Geometry: final body of the model. Coordinates: model frame, mm. A direction names the side the tool comes from. Give positions to 0.01 mm unless a question says otherwise; leave off trailing zeros. Write each loop counter-clockwise with the first axis right and the second up, starting at its lowest first coordinate (ties: lowest second). Pieces come first, ordered by that corner, then holes. Notation, with made-up numbers: M 37,51.5 L 90,51.5 A22 ccw 90,71.5 Z; hole C 74,77 d9. An arc over 180 degrees is marked long. Use a Markdown table: item, result. Add a question column.
(1) Draft query along X for faces 1 (the flat face through (0, 1, -23)), 2 (the flat face through (42, 0, -28)), 3 (the flat face through (72.4, 1, -42)). Return one class per face: released by +X, released by -X, zero draft, split by the parting line, or undercut.
(2) Pin query (flat end, axial travel): pin 1 Ø0.6 at (x, y) = (11.5, 1) entering from +Z; pin 2 Ø1.8 at (x, z) = (77.4, -42.5) entering from +Y (1 decimal). Return the tip coordinate at first contact, or that it passes through.
(3) Cut plane D-D (y = 1.35). State how many separate pieces and enclosed holes the cut face has, plus the area to 3 significant figures.
(4) Reachability of faces 4 (the flat face through (82.4, 1, -3)), 5 (the flat face through (4, 1, -43)), 6 (the flat face through (83, 1, -45)) from +Z, -Z, +X, -X, +Y, -Y: full face, straight path, thin tool, end or side. Return the list, or none.
(5) Cut plane C-C (x = 44). Output: boundary loops of the cut face in (y, z).
(6) Cut plane A-A (x = 77.4). Output: boundary loops of the cut face in (y, z), plus the area to 3 significant figures.
(7) Cut plane B-B (z = -42.5). Output: boundary loops of the cut face in (x, y), plus the area to 3 significant figures.
(8) Material intervals for L1, parallel to Z at x = 77.4, y = 1.05; L2, parallel to X at y = 1.1, z = -23; L3, parallel to X at y = 0.1, z = -24, sorted ascending.
```python
from build123d import *

# Parameters (mm, degrees)
SKETCH1_R           = 1.5
BOSS_EXTRUDE1_DEPTH = 2
SKETCH2_W           = 8.75
SKETCH2_H           = 3.4
CUT_EXTRUDE1_DEPTH  = 10
FILLET1_R           = 1.3


with BuildPart() as part:
    # Sketch1 → Boss-Extrude1 (new body)
    with BuildSketch(Plane(origin=(0, 0, 0), x_dir=(1, 0, 0), z_dir=(0, 1, 0))):
        Polygon((0, 0), (2, 0), (2, 5), (4, 5), (4, 0), (10, 0), (10, 5), (12, 5), (12, 0), (72.4, 0), (72.4, 5), (74.4, 5), (74.4, 0), (80.4, 0), (80.4, 5), (82.4, 5), (82.4, 0), (84.4, 0), (84.4, 45), (82.4, 45), (82.4, 40), (80.4, 40), (80.4, 45), (74.4, 45), (74.4, 40), (72.4, 40), (72.4, 45), (12, 45), (12, 40), (10, 40), (10, 45), (4, 45), (4, 40), (2, 40), (2, 45), (0, 45), align=None)
        with Locations(Location((7, 42.5, 0), (0, 0, 270))):
            Circle(SKETCH1_R, mode=Mode.SUBTRACT)
        with Locations(Location((77.4, 42.5, 0), (0, 0, 90))):
            Circle(SKETCH1_R, mode=Mode.SUBTRACT)
        with Locations(Location((7, 2.5, 0), (0, 0, 90))):
            Circle(SKETCH1_R, mode=Mode.SUBTRACT)
        with Locations(Location((77.4, 2.5, 0), (0, 0, 270))):
            Circle(SKETCH1_R, mode=Mode.SUBTRACT)
    extrude(amount=BOSS_EXTRUDE1_DEPTH)

    # Sketch2 → Cut-Extrude1 (cut)
    with BuildSketch(Plane(origin=(0, 2, 0), x_dir=(1, 0, 0), z_dir=(0, 1, 0))):
        with Locations((42.2, 22.5)):
            Rectangle(SKETCH2_W, SKETCH2_H)
    extrude(amount=-CUT_EXTRUDE1_DEPTH, mode=Mode.SUBTRACT)

    # Fillet1
    fillet1_edges = [part.edges().sort_by_distance(p)[0] for p in [
        (46.575, 1, -24.2),
        (46.575, 1, -20.8),
        (37.825, 1, -20.8),
        (37.825, 1, -24.2),
    ]]
    fillet(fillet1_edges, radius=FILLET1_R)


solid = part.part
```
Answer list:
| question | item | result |
|---|---|---|
| 1 | face 1 | released by -X |
| 1 | face 2 | zero draft |
| 1 | face 3 | undercut |
| 2 | pin 1 | z = -5 |
| 2 | pin 2 | through |
| 3 | separate pieces | 1 |
| 3 | enclosed holes | 5 |
| 3 | area | 3,660 mm² |
| 4 | face 4 | +Z, +Y, -Y |
| 4 | face 5 | -Z, +Y, -Y |
| 4 | face 6 | -Z, +X, -X, +Y, -Y |
| 5 | outline | M 0,-45 L 2,-45 L 2,-24.2 L 0,-24.2 Z; M 0,-20.8 L 2,-20.8 L 2,0 L 0,0 Z |
| 6 | outline | M 0,-45 L 2,-45 L 2,-44 L 0,-44 Z; M 0,-41 L 2,-41 L 2,-4 L 0,-4 Z; M 0,-1 L 2,-1 L 2,0 L 0,0 Z |
| 6 | area | 78.0 mm² |
| 7 | outline | M 0,0 L 2,0 L 2,2 L 0,2 Z; M 4,0 L 5.5,0 L 5.5,2 L 4,2 Z; M 8.5,0 L 10,0 L 10,2 L 8.5,2 Z; M 12,0 L 72.4,0 L 72.4,2 L 12,2 Z; M 74.4,0 L 75.9,0 L 75.9,2 L 74.4,2 Z; M 78.9,0 L 80.4,0 L 80.4,2 L 78.9,2 Z; M 82.4,0 L 84.4,0 L 84.4,2 L 82.4,2 Z |
| 7 | area | 141 mm² |
| 8 | L1 | -45 to -44, -41 to -4, -1 to 0 |
| 8 | L2 | 0 to 37.83, 46.57 to 84.4 |
| 8 | L3 | 0 to 38.43, 45.97 to 84.4 |
